Autodesk Inventor part; units mm, degrees
ref_plane "YZ Plane" through (0, 0, 0) normal (1, 0, 0) x (0, 1, 0)
ref_plane "XZ Plane" through (0, 0, 0) normal (0, 1, 0) x (-1, 0, 0)
ref_plane "XY Plane" through (0, 0, 0) normal (0, 0, 1) x (1, 0, 0)
sketch "Sketch1" plane through (0, 0, 0) normal (1, 0, 0) x (0, 1, 0)
  line L0 (5.2514, 14.5134) -> (-14.7486, 14.5134)
  line L1 (-14.7486, 14.5134) -> (-14.7486, -30.4866)
  line L2 (-14.7486, -30.4866) -> (5.2514, -30.4866)
  line L3 (5.2514, -30.4866) -> (5.2514, 14.5134)
  line L4 (3.2514, 12.5134) -> (-12.7486, 12.5134)
  line L5 (-12.7486, 12.5134) -> (-12.7486, -28.4866)
  line L6 (-12.7486, -28.4866) -> (3.2514, -28.4866)
  line L7 (3.2514, -28.4866) -> (3.2514, 12.5134)
  circle A0 centre (-4.7486, -20.4866) radius 8
  line L8 (3.2514, -7.9866) -> (-3.9727, -7.9866)
  circle A1 centre (-4.7486, 4.5134) radius 8
  point P0 (0, 0)
  dimension "d0" = 20
  dimension "d1" = 45
extrude "Extrusion1" add sketch "Sketch1" along normal blind 1.5 contours L3 L2 L1 L0 | L7 A1 L4 | A1 L5 L4 | A1 | L7 A0 L5 A1 | A0 L6 L5 | A0 | L7 L6 A0
extrude "Extrusion2" add sketch "Sketch1" along normal blind 13.5 contours A1 | A0
properties part number "HCSR04"
For this review, take the finished solid that the model builds, in its own axes (mm). A direction names the side the tool comes from. Give positions to 0.01 mm unless a question says otherwise; leave off trailing zeros. Order: outer loops, then holes, each group sorted by start corner. A loop starts at its lowest first (then second) coordinate and runs counter-clockwise, first axis right, second up. Notation, with made-up numbers: (35.25, 8.5) - (69.25, 8.5) arc R16 ccw to (69.25, 20.5) - close; hole circle Ø4 at (35, -0.5). An arc over 180 degrees is marked (long way). Answer as a JSON object with one key per item and string values. Group by question number.
Item 1: Machinability: for faces 1 (the flat face through (13.5, -5, -20)), 2 (the cylindrical face through (7.4, -0.4, -27.2)), which of the approach directions +Z, -Z, +X, -X, +Y, -Y give a long, thin tool a straight path to every point of the face, cutting with its end or side? Answer none if there is none.
Item 2: Take a section at D-D on z = -6.5. Give the boundary of the cut face in (x, y).
Item 3: Draft analysis for pull direction Z (two halves, no side actions). For faces 3 (the cylindrical face through (7.42, 2.88, 2.11)), 4 (the flat face through (1, 5.251, -8)), 5 (the flat face through (1, -5, 14.513)), state which applies: pulls with the +Z half, pulls with the -Z half, needs draft (parallel to the pull), parting line crosses it, or undercut.
Item 4: Take a section at C-C on x = 2.5. Give the boundary of the cut face in (y, z).
Item 5: Take a section at B-B on z = -16. Give the boundary of the cut face in (x, y), and give its area (3 significant figures).
Item 6: Clearance check with flat-ended pins moving along their axes: pin 1 Ø5 at (x, z) = (2.5, 1.5) entering from +Y; pin 2 Ø1.5 at (x, y) = (10, -7.5) entering from -Z; pin 3 Ø4 at (x, z) = (8.5, -4.5) entering from -Y; pin 4 Ø2 at (x, y) = (7, -3) entering from +Z. State where each tip first meets the part, or that it passes through.
Item 7: Wall thickness on line 1 along Z through (x, y) = (10.5, 2.5); line 2 along Z through (x, y) = (6, -11); line 3 along X through (y, z) = (-2, -4): over which ranges is each line inside the solid? List them lowest first.
Item 8: Take a section at A-A on y = -9.5. Give the boundary of the cut face in (x, z).
Reported:
{
 "1": {"face 1": "+Z, -Z, +X, +Y, -Y", "face 2": "+X"},
 "2": {"outline": "(0, -14.75) - (1.5, -14.75) - (1.5, 5.25) - (0, 5.25) - close"},
 "3": {"face 3": "undercut", "face 4": "needs draft", "face 5": "pulls with the +Z half"},
 "4": {"outline": "circle Ø16 at (-4.75, -20.49); circle Ø16 at (-4.75, 4.51)"},
 "5": {"outline": "(0, -14.75) - (1.5, -14.75) - (1.5, -11.37) - (13.5, -11.37) - (13.5, 1.87) - (1.5, 1.87) - (1.5, 5.25) - (0, 5.25) - close", "area": "189 mm^2"},
 "6": {"pin 1": "y = 5.25", "pin 2": "z = -28.23", "pin 3": "y = -8.6", "pin 4": "z = 12.48"},
 "7": {"line 1": "-23.87 to -17.1, 1.13 to 7.9", "line 2": "-25.48 to -15.49, -0.48 to 9.51", "line 3": "0 to 1.5"},
 "8": {"outline": "(0, -30.49) - (1.5, -30.49) - (1.5, -26.92) - (13.5, -26.92) - (13.5, -14.05) - (1.5, -14.05) - (1.5, -1.92) - (13.5, -1.92) - (13.5, 10.95) - (1.5, 10.95) - (1.5, 14.51) - (0, 14.51) - close"}
}
